from build123d import *

# Parameters (mm, degrees)
V_SLOT_START                           = -5.085646751
V_SLOT_20X20X500_LINEAR_RAIL_OUTLINE_R = 2.1
V_SLOT_20X20X500_LINEAR_RAIL_DEPTH     = 500
SKETCH1_W                              = 20
SKETCH1_H                              = 335
CUT_EXTRUDE1_DEPTH                     = 497.589794047


# Read off the part's stored shape, not the designer's step: V-Slot 20x20x500 Linear Rail
with BuildPart() as part:
    # V-Slot 20x20x500 Linear Rail outline → V-Slot 20x20x500 Linear Rail (new body)
    with BuildSketch(Plane.XY.offset(V_SLOT_START)):
        with BuildLine():
            Line((-21.613469268, 24.462926439), (-21.613469268, 27.092266268))
            Line((-21.613469268, 27.092266268), (-21.823469268, 27.302266268))
            Line((-21.823469268, 27.302266268), (-21.613469268, 27.512266268))
            Line((-21.613469268, 27.512266268), (-21.613469268, 30.141606096))
            Line((-21.613469268, 30.141606096), (-18.952809096, 32.802266268))
            Line((-18.952809096, 32.802266268), (-17.313469268, 32.802266268))
            Line((-17.313469268, 32.802266268), (-17.313469268, 30.427266268))
            Line((-17.313469268, 30.427266268), (-16.968469268, 30.427266268))
            Line((-16.968469268, 30.427266268), (-15.513469268, 31.882266268))
            Line((-15.513469268, 31.882266268), (-15.513469268, 36.802266268))
            ThreePointArc((-15.513469268, 36.802266268), (-15.659915878, 37.155819658), (-16.013469268, 37.302266268))
            Line((-16.013469268, 37.302266268), (-20.933469268, 37.302266268))
            Line((-20.933469268, 37.302266268), (-22.388469268, 35.847266268))
            Line((-22.388469268, 35.847266268), (-22.388469268, 35.502266268))
            Line((-22.388469268, 35.502266268), (-20.013469268, 35.502266268))
            Line((-20.013469268, 35.502266268), (-20.013469268, 33.862926439))
            Line((-20.013469268, 33.862926439), (-22.67412944, 31.202266268))
            Line((-22.67412944, 31.202266268), (-25.303469268, 31.202266268))
            Line((-25.303469268, 31.202266268), (-25.513469268, 30.992266268))
            Line((-25.513469268, 30.992266268), (-25.723469268, 31.202266268))
            Line((-25.723469268, 31.202266268), (-28.352809096, 31.202266268))
            Line((-28.352809096, 31.202266268), (-31.013469268, 33.862926439))
            Line((-31.013469268, 33.862926439), (-31.013469268, 35.502266268))
            Line((-31.013469268, 35.502266268), (-28.638469268, 35.502266268))
            Line((-28.638469268, 35.502266268), (-28.638469268, 35.847266268))
            Line((-28.638469268, 35.847266268), (-30.093469268, 37.302266268))
            Line((-30.093469268, 37.302266268), (-35.013469268, 37.302266268))
            ThreePointArc((-35.013469268, 37.302266268), (-35.367022659, 37.155819658), (-35.513469268, 36.802266268))
            Line((-35.513469268, 36.802266268), (-35.513469268, 31.882266268))
            Line((-35.513469268, 31.882266268), (-34.058469268, 30.427266268))
            Line((-34.058469268, 30.427266268), (-33.713469268, 30.427266268))
            Line((-33.713469268, 30.427266268), (-33.713469268, 32.802266268))
            Line((-33.713469268, 32.802266268), (-32.07412944, 32.802266268))
            Line((-32.07412944, 32.802266268), (-29.413469268, 30.141606096))
            Line((-29.413469268, 30.141606096), (-29.413469268, 27.512266268))
            Line((-29.413469268, 27.512266268), (-29.203469268, 27.302266268))
            Line((-29.203469268, 27.302266268), (-29.413469268, 27.092266268))
            Line((-29.413469268, 27.092266268), (-29.413469268, 24.462926439))
            Line((-29.413469268, 24.462926439), (-32.07412944, 21.802266268))
            Line((-32.07412944, 21.802266268), (-33.713469268, 21.802266268))
            Line((-33.713469268, 21.802266268), (-33.713469268, 24.177266268))
            Line((-33.713469268, 24.177266268), (-34.058469268, 24.177266268))
            Line((-34.058469268, 24.177266268), (-35.513469268, 22.722266268))
            Line((-35.513469268, 22.722266268), (-35.513469268, 17.802266268))
            ThreePointArc((-35.513469268, 17.802266268), (-35.367022659, 17.448712877), (-35.013469268, 17.302266268))
            Line((-35.013469268, 17.302266268), (-30.093469268, 17.302266268))
            Line((-30.093469268, 17.302266268), (-28.638469268, 18.757266268))
            Line((-28.638469268, 18.757266268), (-28.638469268, 19.102266268))
            Line((-28.638469268, 19.102266268), (-31.013469268, 19.102266268))
            Line((-31.013469268, 19.102266268), (-31.013469268, 20.741606096))
            Line((-31.013469268, 20.741606096), (-28.352809096, 23.402266268))
            Line((-28.352809096, 23.402266268), (-25.723469268, 23.402266268))
            Line((-25.723469268, 23.402266268), (-25.513469268, 23.612266268))
            Line((-25.513469268, 23.612266268), (-25.303469268, 23.402266268))
            Line((-25.303469268, 23.402266268), (-22.67412944, 23.402266268))
            Line((-22.67412944, 23.402266268), (-20.013469268, 20.741606096))
            Line((-20.013469268, 20.741606096), (-20.013469268, 19.102266268))
            Line((-20.013469268, 19.102266268), (-22.388469268, 19.102266268))
            Line((-22.388469268, 19.102266268), (-22.388469268, 18.757266268))
            Line((-22.388469268, 18.757266268), (-20.933469268, 17.302266268))
            Line((-20.933469268, 17.302266268), (-16.013469268, 17.302266268))
            ThreePointArc((-16.013469268, 17.302266268), (-15.659915877, 17.448712878), (-15.513469268, 17.802266268))
            Line((-15.513469268, 17.802266268), (-15.513469268, 22.722266268))
            Line((-15.513469268, 22.722266268), (-16.968469268, 24.177266268))
            Line((-16.968469268, 24.177266268), (-17.313469268, 24.177266268))
            Line((-17.313469268, 24.177266268), (-17.313469268, 21.802266268))
            Line((-17.313469268, 21.802266268), (-18.952809096, 21.802266268))
            Line((-18.952809096, 21.802266268), (-21.613469268, 24.462926439))
        make_face()
        with Locations((-25.513469268, 27.302266268)):
            Circle(V_SLOT_20X20X500_LINEAR_RAIL_OUTLINE_R, mode=Mode.SUBTRACT)
    extrude(amount=V_SLOT_20X20X500_LINEAR_RAIL_DEPTH)

    # Sketch1 → Cut-Extrude1 (cut, through all)
    with BuildSketch(Plane(origin=(0, 37.302266268, 0), x_dir=(1, 0, 0), z_dir=(0, 1, 0))):
        with Locations((-25.513469268, -327.414353249)):
            Rectangle(SKETCH1_W, SKETCH1_H)
    extrude(amount=-CUT_EXTRUDE1_DEPTH, mode=Mode.SUBTRACT)


solid = part.part
Could you check a few things on this model? Use its own coordinates, in mm. A direction names the side the tool comes from. Give positions to 0.01 mm unless a question says otherwise; leave off trailing zeros. Return JSON: item names as keys, results as strings.
Item 1: We'd pull the mould along X, two halves only. Please class faces 5 (the flat face through (-18, 37.302, 76)), 6 (the flat face through (-15.513, 20, 76)), 7 (the flat face through (-21.325, 32.551, 76.259)), 8 (the flat face through (-29.413, 29, 76)): +X half, -X half, draft (parallel to the pull), parting line (faces both ways), or undercut.
Geometry results:
{"face 5": "draft", "face 6": "+X half", "face 7": "undercut", "face 8": "-X half"}
Item 2: I need wall thicknesses on L1, parallel to X at y = 19, z = 84.5; L2, parallel to X at y = 20.5, z = 24; L3, parallel to X at y = 31.25, z = 48. Which ranges of each line are inside material? Lowest first, please. Write a range as from..to.
Geometry results:
{"L1": "x = -35.51..-28.64, -22.39..-15.51", "L2": "x = -35.51..-31.01, -20.01..-15.51", "L3": "x = -34.88..-33.71, -30.52..-28.4, -22.63..-20.51, -17.31..-16.15"}
Item 3: I'm going to push flat-ended pins straight in: pin 1 (1 mm diameter, centred on y = 27, z = 79.5, fed in from -X); pin 2 (2 mm diameter, centred on y = 28.5, z = 110, fed in from +X); pin 3 (1 mm diameter, centred on x = -25, z = 139, fed in from +Y). Where does each tip first touch, or does it pass through?
Geometry results:
{"pin 1": "stops at x = -29.41", "pin 2": "stops at x = -21.61", "pin 3": "stops at y = 31.2"}
Item 4: Which directions (+Z, -Z, +X, -X, +Y, -Y) give clear straight access to the entire face, cutting with the end or side of a thin tool? Please do faces 1 (the flat face through (-27, 31.202, 76)), 2 (the flat face through (-27, 23.402, 76)), 3 (the flat face through (-29.702, 22.053, 76.259)), 4 (the flat face through (-21.613, 26, 76)).
Geometry results:
{"face 1": "+Z, -Z, +Y", "face 2": "+Z, -Z, -Y", "face 3": "+Z, -Z", "face 4": "+Z, -Z, +X"}
